Build history of the part. All positions in model axes, mm. A direction names the side the tool comes from. Give positions to 0.01 mm unless a question says otherwise; leave off trailing zeros. Loops run counter-clockwise (first coordinate to the right, second up) from the corner with the lowest first, then second, coordinate; pieces in that order, holes last.
1) Band-saw the part on A-A on z = 0.15. List the corners of the cut face in (x, y).
2) Wall check: line 1 (Z direction, x = -1.5, y = 1.5); line 2 (Y direction, x = 1.15, z = 0.15); line 3 (X direction, y = -2.5, z = 0.15). Give the ranges that are in metal, low to high.
3) Band-saw the part on D-D on y = -5. List the corners of the cut face in (x, z).
4) 3-axis set-ups, long thin cutter, end or side, ignore diameter. For faces 1 (the flat face through (0, -1, 0)), 2 (the flat face through (-2.2, -1.4, 0.2)): which of +Z, -Z, +X, -X, +Y, -Y reach the whole face in a straight line?
```python
from build123d import *

# Parameters (mm, degrees)
BOSS_EXTRUDE1_DEPTH = 0.2
SKETCH2_R           = 2.206807536
BOSS_EXTRUDE2_DEPTH = 0.25
BOSS_EXTRUDE3_DEPTH = 0.06
SKETCH5_R           = 0.3
CUT_EXTRUDE1_DEPTH  = 1.26


with BuildPart() as part:
    # Sketch1 → Boss-Extrude1 (new body)
    with BuildSketch(Plane.XY):
        with BuildLine():
            Line((-2.8, -6.25), (2.8, -6.25))
            Line((2.8, -6.25), (2.8, -2.484625193))
            ThreePointArc((2.8, -2.484625193), (2.861380635, -1.801298833), (3.043557337, -1.139850312))
            ThreePointArc((3.043557337, -1.139850312), (0, 3.25), (-3.043557337, -1.139850312))
            ThreePointArc((-3.043557337, -1.139850312), (-2.861380635, -1.801298833), (-2.8, -2.484625193))
            Line((-2.8, -2.484625193), (-2.8, -6.25))
        make_face()
    extrude(amount=BOSS_EXTRUDE1_DEPTH)

    # Sketch2 → Boss-Extrude2 (add)
    with BuildSketch(Plane(origin=(0, 0, 0), x_dir=(-1, 0, 0), z_dir=(0, 0, -1))):
        Circle(SKETCH2_R)
    extrude(amount=-BOSS_EXTRUDE2_DEPTH)

    # Sketch3 → Boss-Extrude3 (add)
    with BuildSketch(Plane.XY.offset(0.2)):
        with BuildLine():
            Line((0.870696458, -1.846445486), (0.870696458, -3.07534158))
            Line((0.870696458, -3.07534158), (2.15, -4.550780247))
            Line((2.15, -4.550780247), (2.15, -6.25))
            Line((2.15, -6.25), (0.337052097, -6.25))
            Line((0.337052097, -6.25), (0.337052097, -2.013422245))
            ThreePointArc((0.337052097, -2.013422245), (0, -2.041439016), (-0.337052097, -2.013422245))
            Line((-0.337052097, -2.013422245), (-0.337052097, -6.25))
            Line((-0.337052097, -6.25), (-2.15, -6.25))
            Line((-2.15, -6.25), (-2.15, -4.550780247))
            Line((-2.15, -4.550780247), (-0.870696458, -3.07534158))
            Line((-0.870696458, -3.07534158), (-0.870696458, -1.846445486))
            ThreePointArc((-0.870696458, -1.846445486), (0, 2.041439016), (0.870696458, -1.846445486))
        make_face()
        with BuildLine():
            Line((-0.8, 1.15), (1.081903016, 1.15))
            ThreePointArc((1.081903016, 1.15), (-0.385798466, 1.531069456), (-1.497669568, 0.5))
            Line((-1.497669568, 0.5), (1.15, 0.5))
            Line((1.15, 0.5), (1.15, 0.15))
            Line((1.15, 0.15), (-1.571786925, 0.15))
            ThreePointArc((-1.571786925, 0.15), (-1.54152787, -0.341622545), (-1.361254618, -0.8))
            Line((-1.361254618, -0.8), (0.8, -0.8))
            Line((0.8, -0.8), (0.8, -1.15))
            Line((0.8, -1.15), (-1.081903016, -1.15))
            ThreePointArc((-1.081903016, -1.15), (0.385798466, -1.531069456), (1.497669568, -0.5))
            Line((1.497669568, -0.5), (-1.15, -0.5))
            Line((-1.15, -0.5), (-1.15, -0.15))
            Line((-1.15, -0.15), (1.571786925, -0.15))
            ThreePointArc((1.571786925, -0.15), (1.540204935, 0.347538335), (1.355071738, 0.810428727))
            Line((1.355071738, 0.810428727), (1.355071738, 0.8))
            Line((1.355071738, 0.8), (-0.8, 0.8))
            Line((-0.8, 0.8), (-0.8, 1.15))
        make_face(mode=Mode.SUBTRACT)
    extrude(amount=BOSS_EXTRUDE3_DEPTH)

    # Sketch5 → Cut-Extrude1 (cut, through all)
    with BuildSketch(Plane.XY.offset(0.26)):
        with Locations((-1.15, -5.75)):
            Circle(SKETCH5_R)
        with Locations((1.15, -5.75)):
            Circle(SKETCH5_R)
    extrude(amount=-CUT_EXTRUDE1_DEPTH, mode=Mode.SUBTRACT)


solid = part.part
```
Findings below:
1. outline: (-3.04, -1.14) arc R3.83 cw to (-2.8, -2.48) - (-2.8, -6.25) - (2.8, -6.25) - (2.8, -2.48) arc R3.83 cw to (3.04, -1.14) arc R3.25 ccw (long way) to start; hole circle Ø0.6 at (-1.15, -5.75); hole circle Ø0.6 at (1.15, -5.75)
2. line 1: z = 0 to 0.25
2. line 2: y = -6.25 to -6.05, -5.45 to 3.04
2. line 3: x = -2.8 to 2.8
3. outline: (-2.8, 0) - (2.8, 0) - (2.8, 0.2) - (2.15, 0.2) - (2.15, 0.26) - (0.34, 0.26) - (0.34, 0.2) - (-0.34, 0.2) - (-0.34, 0.26) - (-2.15, 0.26) - (-2.15, 0.2) - (-2.8, 0.2) - close
4. face 1: -Z, +X, -X, +Y, -Y
4. face 2: +Z
